```python
from build123d import *

# Parameters (mm, degrees)
F1_DEPTH = 100
F3_D     = 16


with BuildPart() as f1:
    # F0 (on Front) → F1 (new body)
    with BuildSketch(Plane.XZ):
        with BuildLine():
            Line((34.5, 0), (44.5, 0))
            ThreePointArc((44.5, 0), (38.02781, 23.111376), (20.493902, 39.5))
            Line((20.493902, 39.5), (-20.493902, 39.5))
            ThreePointArc((-20.493902, 39.5), (-38.02781, 23.111376), (-44.5, 0))
            Line((-44.5, 0), (-34.5, 0))
            ThreePointArc((-34.5, 0), (0, 34.5), (34.5, 0))
        make_face()
    extrude(amount=F1_DEPTH)

    # F3 (through all)
    with Locations(Plane.XY.offset(39.5)):
        with Locations((0, -50)):
            Hole(F3_D / 2)


solid = f1.part
```
Input: part model. Units: mm. Frame: model coordinates. Coordinates: 2 decimals unless noted, no trailing zeros. Loops run counter-clockwise (first coordinate to the right, second up) from the corner with the lowest first, then second, coordinate; pieces in that order, holes last. Notation, with made-up numbers: M 78,1 L 84,1 A16 ccw 84,26 Z; hole C 15,76 d6. An arc over 180 degrees is marked long. Use a Markdown table: item, result. Add a question column.
1) Section C-C, the plane x = 0. Return the cut outline in (y, z).
2) Section A-A, the plane y = -50. Return the cut outline in (x, z), plus the area to 3 significant figures.
3) Pin query (flat end, axial travel): P1, Ø21, axis at x = 0, y = -50, coming from the +Z side; P2, Ø1, axis at x = -4.5, y = -40.5, coming from the -Z side; P3, Ø4, axis at y = -14.5, z = 6.5, coming from the +X side. Return the tip coordinate at first contact, or that it passes through.
4) Draft query along X for faces 1 (the flat face through (0, -100, 36)), 2 (the cylindrical face through (-12.51, -49.3, 32.15)), 3 (the cylindrical face through (-37.85, -49.3, 23.4)), 4 (the cylindrical face through (38.203, -49.3, 22.82)). Return one class per face: +X half, -X half, draft (parallel to the pull), parting line (faces both ways), or undercut.
5) Section D-D, the plane y = -74. Return the cut outline in (x, z).
6) Section B-B, the plane z = 30.5. Return the cut outline in (x, y), plus the area to 3 significant figures.
7) Line query: L1, parallel to Y at x = 0, z = 37.4; L2, parallel to Z at x = -0.5, y = -35; L3, parallel to X at y = -83, z = 12.5. Output: solid intervals per line, ascending. Write a range as from..to.
Answer below:
| question | item | result |
|---|---|---|
| 1 | outline | M -100,34.5 L -58,34.5 L -58,39.5 L -100,39.5 Z; M -42,34.5 L 0,34.5 L 0,39.5 L -42,39.5 Z |
| 2 | outline | M -44.5,0 L -34.5,0 A34.5 cw -8,33.56 L -8,39.5 L -20.49,39.5 A44.5 ccw Z; M 8,33.56 A34.5 cw 34.5,0 L 44.5,0 A44.5 ccw 20.49,39.5 L 8,39.5 Z |
| 2 | area | 1,020 mm2 |
| 3 | P1 | z = 39.5 |
| 3 | P2 | z = 34.14 |
| 3 | P3 | x = 44.27 |
| 4 | face 1 | draft |
| 4 | face 2 | undercut |
| 4 | face 3 | -X half |
| 4 | face 4 | +X half |
| 5 | outline | M -44.5,0 L -34.5,0 A34.5 cw 34.5,0 L 44.5,0 A44.5 ccw 20.49,39.5 L -20.49,39.5 A44.5 ccw Z |
| 6 | outline | M -32.4,-100 L -16.12,-100 L -16.12,0 L -32.4,0 Z; M 16.12,-100 L 32.4,-100 L 32.4,0 L 16.12,0 Z |
| 6 | area | 3,260 mm2 |
| 7 | L1 | -100..-58, -42..0 |
| 7 | L2 | 34.5..39.5 |
| 7 | L3 | -42.71..-32.16, 32.16..42.71 |
